Autodesk Inventor part; units mm, degrees
ref_plane "YZ Plane" through (0, 0, 0) normal (1, 0, 0) x (0, 1, 0)
ref_plane "XZ Plane" through (0, 0, 0) normal (0, 1, 0) x (-1, 0, 0)
ref_plane "XY Plane" through (0, 0, 0) normal (0, 0, 1) x (1, 0, 0)
sketch "Sketch1" plane through (0, 0, 0) normal (0, 0, 1) x (1, 0, 0)
  line L0 (-76.2, 25.4) -> (76.2, 25.4) construction
  line L1 (76.2, 25.4) -> (76.2, -25.4) construction
  line L2 (76.2, -25.4) -> (-76.2, -25.4) construction
  line L3 (-76.2, -25.4) -> (-76.2, 25.4) construction
  line L4 (-76.2, 25.4) -> (76.2, -25.4) construction
  line L5 (76.2, 25.4) -> (-76.2, -25.4) construction
  line L6 (63.5, 17.4625) -> (63.5, -17.4625) construction
  line L7 (9.525, 15.875) -> (41.275, 15.875) construction
  line L8 (41.275, 15.875) -> (41.275, -15.875) construction
  line L9 (41.275, -15.875) -> (9.525, -15.875) construction
  line L10 (9.525, -15.875) -> (9.525, 15.875) construction
  line L11 (9.525, 15.875) -> (41.275, -15.875) construction
  line L12 (41.275, 15.875) -> (9.525, -15.875) construction
  line L13 (76.2, 101.6) -> (187.452, 101.6) construction
  line L14 (187.452, 101.6) -> (187.452, -25.4) construction
  line L15 (187.452, -25.4) -> (76.2, -25.4) construction
  line L16 (76.2, -25.4) -> (76.2, 101.6) construction
  line L17 (76.2, 101.6) -> (187.452, -25.4) construction
  line L18 (187.452, 101.6) -> (76.2, -25.4) construction
  point P0 (0, 0)
  point P1 (63.5, 0)
  point P2 (25.4, 0)
  point P3 (50.8, 0)
  point P4 (0, 0)
  point P5 (9.525, 0)
  point P6 (-12.7, 17.4625)
  point P7 (-12.7, -17.4625)
  point P8 (-25.4, 0)
  point P9 (-38.1, 17.4625)
  point P10 (-38.1, -17.4625)
  point P11 (-50.8, 0)
  point P12 (-63.5, 17.4625)
  point P13 (-63.5, -17.4625)
  point P14 (131.826, 38.1)
  dimension "d0" = 152.4
  dimension "d1" = 50.8
  dimension "d2" = 34.925
  dimension "d3" = 12.7
  dimension "d4" = 31.75
  dimension "d5" = 31.75
  dimension "d6" = 34.925
  dimension "d7" = 25.4
  dimension "d8" = 9.525
  dimension "d9" = 12.7
  dimension "d10" = 12.7
  dimension "d11" = 12.7
  dimension "d12" = 12.7
  dimension "d13" = 12.7
  dimension "d14" = 111.252
  dimension "d15" = 127
  dimension "d16" = 76.2
sketch "Sketch2" plane through (0, 0, 0) normal (0, 0, 1) x (1, 0, 0)
  line L0 (63.5, 17.4625) -> (63.5, -17.4625) construction
  line L1 (76.2, 25.4) -> (76.2, -25.4) construction
  line L2 (76.2, -25.4) -> (76.2, 101.6) construction
  line L3 (187.452, -25.4) -> (76.2, -25.4) construction
  line L4 (187.452, 101.6) -> (187.452, -25.4) construction
  line L5 (76.2, 101.6) -> (187.452, -25.4) construction
  line L6 (187.452, 101.6) -> (76.2, -25.4) construction
  line L7 (76.2, 101.6) -> (187.452, 101.6) construction
  line L8 (9.525, 15.875) -> (41.275, 15.875) construction
  line L9 (41.275, 15.875) -> (41.275, -15.875) construction
  line L10 (41.275, -15.875) -> (9.525, -15.875) construction
  line L11 (9.525, -15.875) -> (9.525, 15.875) construction
  line L12 (9.525, 15.875) -> (41.275, -15.875) construction
  line L13 (41.275, 15.875) -> (9.525, -15.875) construction
  line L14 (-76.2, 25.4) -> (76.2, 25.4) construction
  line L15 (76.2, -25.4) -> (-76.2, -25.4) construction
  line L16 (-76.2, 25.4) -> (76.2, -25.4) construction
  line L17 (76.2, 25.4) -> (-76.2, -25.4) construction
  line L18 (-76.2, -25.4) -> (-76.2, 25.4) construction
  line L19 (0, 25.4) -> (0, -25.4)
  line L20 (0, -25.4) -> (-76.2, -25.4)
  line L21 (-76.2, -25.4) -> (-76.2, 25.4)
  line L22 (-76.2, 25.4) -> (25.7652, 154.4619)
  circle A0 centre (44.45, 139.7) radius 14.2875
  circle A1 centre (44.45, 139.7) radius 23.8125 construction
  line L23 (68.2061, 141.338) -> (76.2, 25.4)
  line L24 (76.2, 25.4) -> (76.2, -25.4)
  line L25 (76.2, -25.4) -> (50.8, -25.4)
  line L26 (50.8, -25.4) -> (50.8, 25.4)
  line L27 (50.8, 25.4) -> (0, 25.4)
  arc A2 (68.2061, 141.338) -> (25.7652, 154.4619) centre (44.45, 139.7) ccw
  point P0 (0, 0)
  point P1 (63.5, 0)
  point P2 (131.826, 38.1)
  point P3 (9.525, 0)
  point P4 (0, 0)
  point P5 (25.4, 0)
  point P6 (-63.5, -17.4625)
  point P7 (-63.5, 17.4625)
  point P8 (-50.8, 0)
  point P9 (-38.1, -17.4625)
  point P10 (-38.1, 17.4625)
  point P11 (-25.4, 0)
  point P12 (-12.7, -17.4625)
  point P13 (-12.7, 17.4625)
  point P14 (0, 0)
  point P15 (50.8, 0)
  point P16 (0, 0)
  dimension "d17" = 28.575
  dimension "d18" = 9.525
  dimension "d20" = 9.525
  dimension "d21" = 9.525
  dimension "d31" = 165.1
  dimension "d32" = 19.05
extrude "Extrusion1" add sketch "Sketch2" along normal blind 6.35
hole "Hole1" at (76.2, 101.6, 0) at (131.826, 38.1, 0) at (187.452, -25.4, 0) at (9.525, 0, 0) at (9.525, 15.875, 0) at (41.275, -15.875, 0) at (41.275, 15.875, 0) at (9.525, -15.875, 0) at (25.4, 0, 0) at (-63.5, -17.4625, 0) at (-63.5, 17.4625, 0) at (-50.8, 0, 0) at (-38.1, -17.4625, 0) at (-38.1, 17.4625, 0) at (-25.4, 0, 0) at (-12.7, -17.4625, 0) at (-12.7, 17.4625, 0) at (63.5, 17.4625, 0) at (63.5, -17.4625, 0) direction (0, 0, 1) diameter 5.1054 end through all
fillet "Fillet1" radius 6.604 7 edges at (50.8, 25.4, 3.175) (0, 25.4, 3.175) (0, -25.4, 3.175) (50.8, -25.4, 3.175) (76.2, -25.4, 3.175) (-76.2, -25.4, 3.175) (-76.2, 25.4, 3.175)
sketch "Sketch4" plane through (0, 0, 6.35) normal (0, 0, 1) x (1, 0, 0)
  circle A0 centre (-69.85, 50.8) radius 25.4 construction
  circle A1 centre (-69.85, 50.8) radius 30.48 construction
  circle A2 centre (-69.85, 50.8) radius 9.525
  circle A3 centre (-69.85, 50.8) radius 6.35 construction
  circle A4 centre (-29.0763, 83.185) radius 45.72 construction
  circle A5 centre (63.5, 17.4625) radius 2.5527 construction
  circle A6 centre (-12.7, -17.4625) radius 2.5527 construction
  circle A7 centre (-38.1, 17.4625) radius 2.5527 construction
  circle A8 centre (-50.8, 0) radius 2.5527 construction
  circle A9 centre (-63.5, -17.4625) radius 2.5527 construction
  circle A10 centre (-63.5, 17.4625) radius 2.5527 construction
  circle A11 centre (-38.1, -17.4625) radius 2.5527 construction
  circle A12 centre (-25.4, 0) radius 2.5527 construction
  circle A13 centre (-12.7, 17.4625) radius 2.5527 construction
  circle A14 centre (63.5, -17.4625) radius 2.5527 construction
  circle A15 centre (44.45, 139.7) radius 14.2875 construction
  arc A16 (68.2061, 141.338) -> (25.7652, 154.4619) centre (44.45, 139.7) ccw construction
  line L0 (68.2061, 141.338) -> (76.2, 25.4) construction
  line L1 (76.2, 25.4) -> (76.2, -18.796) construction
  arc A17 (69.596, -25.4) -> (76.2, -18.796) centre (69.596, -18.796) ccw construction
  line L2 (69.596, -25.4) -> (57.404, -25.4) construction
  arc A18 (50.8, -18.796) -> (57.404, -25.4) centre (57.404, -18.796) ccw construction
  line L3 (50.8, -18.796) -> (50.8, 18.796) construction
  arc A19 (50.8, 18.796) -> (44.196, 25.4) centre (44.196, 18.796) ccw construction
  line L4 (44.196, 25.4) -> (6.604, 25.4) construction
  arc A20 (6.604, 25.4) -> (0, 18.796) centre (6.604, 18.796) ccw construction
  line L5 (0, 18.796) -> (0, -18.796) construction
  arc A21 (-6.604, -25.4) -> (0, -18.796) centre (-6.604, -18.796) ccw construction
  line L6 (-6.604, -25.4) -> (-69.596, -25.4) construction
  arc A22 (-76.2, -18.796) -> (-69.596, -25.4) centre (-69.596, -18.796) ccw construction
  line L7 (-76.2, -18.796) -> (-76.2, 23.106) construction
  arc A23 (-74.7779, 27.2) -> (-76.2, 23.106) centre (-69.596, 23.106) ccw
  line L8 (-74.7779, 27.2) -> (25.7652, 154.4619)
  line L9 (76.2, -25.4) -> (-127, -25.4) construction
  line L10 (-127, -25.4) -> (-127, 25.4) construction
  line L11 (-127, 25.4) -> (76.2, 25.4) construction
  line L12 (76.2, 25.4) -> (76.2, -25.4) construction
  circle A24 centre (-29.0763, 83.185) radius 14.2875
  arc A25 (61.8711, 140.9012) -> (30.7478, 150.5254) centre (44.45, 139.7) ccw construction
  line L13 (61.8711, 140.9012) -> (69.85, 25.1813) construction
  line L14 (69.85, 25.1813) -> (69.85, -19.05) construction
  line L15 (69.85, -19.05) -> (57.15, -19.05) construction
  line L16 (57.15, -19.05) -> (57.15, 18.796) construction
  arc A26 (57.15, 18.796) -> (44.196, 31.75) centre (44.196, 18.796) ccw construction
  line L17 (44.196, 31.75) -> (6.604, 31.75) construction
  arc A27 (6.604, 31.75) -> (-6.35, 18.796) centre (6.604, 18.796) ccw construction
  line L18 (-6.35, 18.796) -> (-6.35, -19.05) construction
  line L19 (-6.35, -19.05) -> (-69.85, -19.05) construction
  line L20 (-69.85, -19.05) -> (-69.85, 23.1943) construction
  line L21 (-69.85, 23.1943) -> (30.7478, 150.5254) construction
  circle A28 centre (-29.0763, 83.185) radius 12.7 construction
  circle A29 centre (-80.138, 102.5487) radius 41.91 construction
  circle A30 centre (-80.138, 102.5487) radius 12.7 construction
  circle A31 centre (-55.6558, 151.3634) radius 41.91 construction
  circle A32 centre (-80.138, 102.5487) radius 14.2875
  circle A33 centre (-55.6558, 151.3634) radius 14.2875
  circle A34 centre (-80.138, 102.5487) radius 20.6375 construction
  circle A35 centre (-55.6558, 151.3634) radius 20.6375 construction
  arc A36 (68.2061, 141.338) -> (25.7652, 154.4619) centre (44.45, 139.7) ccw construction
  arc A37 (46.4593, 163.4276) -> (25.7652, 154.4619) centre (44.45, 139.7) ccw
  circle A38 centre (44.45, 139.7) radius 14.2875 construction
  arc A39 (27.8994, 100.6165) -> (37.3281, 181.5416) centre (44.45, 139.7) ccw construction
  circle A40 centre (-80.138, 102.5487) radius 7.366 construction
  line L22 (-76.2, 23.106) -> (-76.2, -18.796) construction
  arc A41 (-100.3289, 50.5378) -> (-76.2, 20.9888) centre (-69.85, 50.8) ccw
  line L23 (-76.2, 20.9888) -> (-76.2, 23.106)
  arc A42 (-58.0297, 165.3106) -> (-61.1726, 138.3355) centre (-55.6558, 151.3634) ccw construction
  line L24 (37.3281, 181.5416) -> (-58.0297, 165.3106) construction
  line L25 (27.8994, 100.6165) -> (-61.1726, 138.3355) construction
  line L26 (-74.1032, 160.6154) -> (-98.5854, 111.8007)
  line L27 (-53.9144, 171.9273) -> (46.4593, 163.4276)
  line L28 (-100.7747, 102.3712) -> (-100.3289, 50.5378)
  arc A43 (-98.5854, 111.8007) -> (-100.7747, 102.3712) centre (-80.138, 102.5487) ccw
  arc A44 (-53.9144, 171.9273) -> (-74.1032, 160.6154) centre (-55.6558, 151.3634) ccw
  point P0 (0, 0)
  point P1 (76.2, 3.302)
  point P2 (76.2, 0)
  point P3 (-44.7862, 54.9187)
  point P4 (-60.885, 74.5653)
  point P5 (-85.9488, 70.4466)
  point P6 (-94.9138, 46.6813)
  point P7 (-78.815, 27.0347)
  point P8 (-53.7512, 31.1534)
  point P9 (-38.81, 72.7262)
  point P10 (-21.1536, 95.0747)
  dimension "d45" = 50.8
  dimension "d46" = 60.96
  dimension "d47" = 19.05
  dimension "d48" = 12.7
  dimension "d49" = 91.44
  dimension "d50" = 6.35
  dimension "d52" = 203.2
  dimension "d53" = 50.8
  dimension "d54" = 76.2
  dimension "d55" = 28.575
  dimension "d56" = 6.35
  dimension "d57" = 25.4
  dimension "d58" = 83.82
  dimension "d59" = 57.785
  dimension "d60" = 25.4
  dimension "d61" = 83.82
  dimension "d64" = 6.35
  dimension "d65" = 6.35
  dimension "d70" = 360
  dimension "d82" = 84.8868
  dimension "d83" = 14.732
  dimension "d86" = 28.2956
  dimension "d92" = 96.7293
  dimension "d93" = 157.4973
  dimension "d94" = 36.3942
  dimension "d95" = 127.9487
extrude "Extrusion3" add sketch "Sketch4" against normal up to surface (6.35 mm away) contours A23 L23 A41 L28 A43 L26 A44 L27 A37 L8 A24 | L8 A24 picked at (-24.9221, 78.7661)
extrude "Extrusion4" cut sketch "Sketch4" against normal through all contours A2 | A24 L8 | L8 A24
hole "Hole2" at (-44.7862, 54.9187, 6.35) at (-60.885, 74.5653, 6.35) at (-85.9488, 70.4466, 6.35) at (-53.7512, 31.1534, 6.35) at (-94.9138, 46.6813, 6.35) direction (0, 0, -1) diameter 5.1054 end through all
fillet "Fillet4" radius 6.604 1 edges at (-76.2, 20.9888, 3.175)
equation "\"off\" = 6.35"
properties part number "CL3-015" material "Aluminum 6061"
Design review of the part built by this model. Coordinates are the model's own, in mm. A direction names the side the tool comes from. Round coordinates to 2 decimals unless told otherwise and drop trailing zeros. Loops run counter-clockwise (first coordinate to the right, second up) from the corner with the lowest first, then second, coordinate; pieces in that order, holes last. Notation, with made-up numbers: (25.5, 32) - (62.5, 32) arc R15 cw to (62.5, 58) - close; hole circle Ø8 at (31, 83.25). An arc over 180 degrees is marked (long way). One line per item, written item: value. Start each with the question number.
1) Consider section C-C on z = 1.25. Give the number of separate pieces and of enclosed holes in the cut face, then the cut area to 3 significant figures.
2) Consider section B-B on y = 95. Give the boundary of the cut face in (x, z).
3) Insertion check: pin 1 Ø2 at (x, z) = (21, 4.5) entering from +Y; pin 2 Ø1.9 at (y, z) = (0.5, 4) entering from -X. Each pin has a flat end and moves straight along its axis. Give the tip position at first contact, or say it passes through.
4) To check wall thickness, follow L1, parallel to X at y = 0.5, z = 0.75; L2, parallel to X at y = 10, z = 4.75; L3, parallel to X at y = 141, z = 3.25. State the ranges of each line that lie inside material, in increasing order. Write a range as from..to.
5) Consider section D-D on y = 37.5. Give the boundary of the cut face in (x, z).
6) Draft analysis for pull direction X (two halves, no side actions). For faces 1 (the flat face through (72.147, 84.181, 3.131)), 2 (the flat face through (-14, 75, 6.35)), 3 (the cylindrical face through (-35.61, -18.02, 3.22)), state which applies: +X half, -X half, draft (parallel to the pull), parting line (faces both ways), or undercut.
7) For faces 4 (the cylindrical face through (52.68, -23.41, 3.22)), 5 (the flat face through (64, -25.4, 3)), list the 3-axis set-ups (+Z, -Z, +X, -X, +Y, -Y) from which the entire face can be reached by the end or side of a thin tool; tool diameter is ignored.
8) Consider section A-A on x = 63.5. Give the boundary of the cut face in (y, z), then the cut area to 3 significant figures.
Reported:
1. separate pieces: 1
1. enclosed holes: 20
1. area: 25,300 mm^2
2. outline: (-100.71, 0) - (-92.27, 0) - (-92.27, 6.35) - (-100.71, 6.35) - close; (-68.01, 0) - (-37.11, 0) - (-37.11, 6.35) - (-68.01, 6.35) - close; (-21.04, 0) - (71.4, 0) - (71.4, 6.35) - (-21.04, 6.35) - close
3. pin 1: stops at y = 165.67
3. pin 2: stops at x = -76.2
4. L1: x = -76.2..-53.3, -48.3..-27.9, -22.9..0, 50.8..76.2
4. L2: x = -76.2..0, 50.8..76.2
4. L3: x = -83.94..-65.49, -45.82..30.22, 58.68..68.23
5. outline: (-97.28, 0) - (75.37, 0) - (75.37, 6.35) - (-97.28, 6.35) - close
6. face 1: +X half
6. face 2: draft
6. face 3: undercut
7. face 4: +Z, -Z, -Y
7. face 5: +Z, -Z, +X, -X, -Y
8. outline: (-25.4, 0) - (-20.02, 0) - (-20.02, 6.35) - (-25.4, 6.35) - close; (-14.91, 0) - (14.91, 0) - (14.91, 6.35) - (-14.91, 6.35) - close; (20.02, 0) - (153.99, 0) - (153.99, 6.35) - (20.02, 6.35) - close
8. area: 1,070 mm^2
